Read the model definition and answer for the solid it produces. Units are mm, in the model's axes. Face numbers are marked on the shaded views. Coordinates: 2 decimals unless noted, no trailing zeros. Loops run counter-clockwise (first coordinate to the right, second up) from the corner with the lowest first, then second, coordinate; pieces in that order, holes last. Notation, with made-up numbers: (49, -10) -> (56, -10) arc R19 cw to (56, -5) -> close; hole circle Ø10 at (61, -32). An arc over 180 degrees is marked (long way). Answer as a JSON object with one key per item and string values. Group by question number.
1) Section B-B, the plane z = 32 is taken. Give the vertices of the cut face in (x, y).
2) Section A-A, the plane x = 20 is taken. Give the vertices of the cut face in (y, z).
3) Consider probe 1 along X at (y, z) = (0.5, 147.5); probe 2 along Z at (x, y) = (34.5, -8.5); probe 3 along Z at (x, y) = (16.5, -7). Determine where each line is inside the solid, lowest interval first. Write a range as [from, to].
4) Section C-C, the plane y = 5 is taken. Give the vertices of the cut face in (x, z), plus the area to 3 significant figures.
5) Flat-ended cylindrical pins translate along their axes: P1, Ø24, axis at x = 28, y = 7, coming from the +Z side; P2, Ø18, axis at y = 0, z = 0, coming from the -X side; P3, Ø3, axis at x = 15.5, y = 9.5, coming from the +Z side; P4, Ø24, axis at x = 28.5, y = -7, coming from the -Z side. Find the tip coordinate at first contact, or state that the pin passes through.
6) Determine the mould class of the marked faces 1, 2, 3 and 4 for opening direction Z: released by +Z, released by -Z, zero draft, split by the parting line, or undercut.
7) Section D-D, the plane y = -14.5 is taken. Give the vertices of the cut face in (x, z).
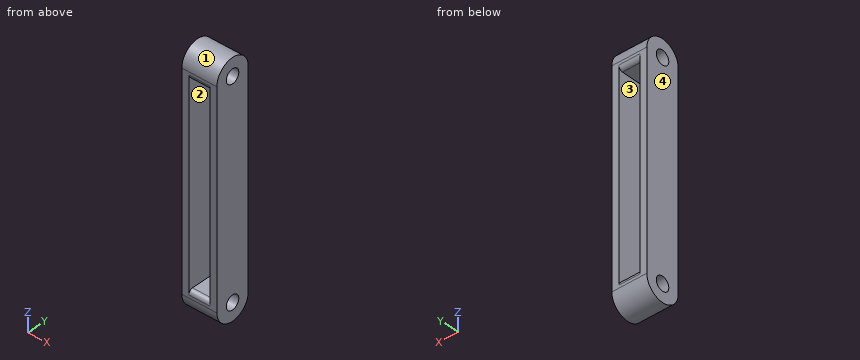
Autodesk Inventor part; units mm, degrees
ref_plane "YZ Plane" through (0, 0, 0) normal (1, 0, 0) x (0, 1, 0)
ref_plane "XZ Plane" through (0, 0, 0) normal (0, 1, 0) x (-1, 0, 0)
ref_plane "XY Plane" through (0, 0, 0) normal (0, 0, 1) x (1, 0, 0)
sketch "Sketch1" plane through (0, 0, 0) normal (1, 0, 0) x (0, 1, 0)
  circle A0 centre (0, 0) radius 25
  line L0 (0, 0) -> (0, 300)
  circle A1 centre (0, 300) radius 25
  circle A2 centre (0, 300) radius 10
  circle A3 centre (0, 0) radius 10
  line L1 (25, 300) -> (25, 0)
  line L2 (-25, 300) -> (-25, 0)
  dimension "d0" = 300
  dimension "d1" = 50
  dimension "d2" = 20
extrude "Extrusion1" add sketch "Sketch1" along normal blind 50
sketch "Sketch2" plane through (0, -25, 0) normal (0, -1, 0) x (1, 0, 0)
  line L0 (0, 0) -> (50, 0)
  line L1 (50, 300) -> (50, 0)
  line L2 (0, 0) -> (50, 0)
  line L3 (50, 0) -> (50, 300)
  line L4 (50, 300) -> (0, 300)
  line L5 (0, 300) -> (0, 0)
  line L6 (10, 10) -> (40, 10)
  line L7 (40, 10) -> (40, 290)
  line L8 (40, 290) -> (10, 290)
  line L9 (10, 290) -> (10, 10)
  dimension "d6" = 10
extrude "Extrusion2" cut sketch "Sketch2" against normal through all contours L9 L8 L7 L6
fillet "Fillet1" radius 6 4 edges at (25, 25, 290) (25, 25, 10) (25, -25, 10) (25, -25, 290)
properties part number "arm1"
Determined:
{
 "1": {"outline": "(0, -25) -> (10, -25) -> (10, 25) -> (0, 25) -> close; (40, -25) -> (50, -25) -> (50, 25) -> (40, 25) -> close"},
 "2": {"outline": "(-25, 0) arc R25 ccw to (25, 0) -> (25, 4) arc R6 ccw to (19, 10) -> (-19, 10) arc R6 ccw to (-25, 4) -> close; (-25, 296) arc R6 ccw to (-19, 290) -> (19, 290) arc R6 ccw to (25, 296) -> (25, 300) arc R25 ccw to (-25, 300) -> close; hole circle Ø20 at (0, 0); hole circle Ø20 at (0, 300)"},
 "3": {"probe 1": "[0, 10], [40, 50]", "probe 2": "[-23.51, -5.27], [5.27, 10], [290, 294.73], [305.27, 323.51]", "probe 3": "[-24, -7.14], [7.14, 10], [290, 292.86], [307.14, 324]"},
 "4": {"outline": "(0, -24.49) -> (50, -24.49) -> (50, -8.66) -> (0, -8.66) -> close; (0, 8.66) -> (50, 8.66) -> (50, 291.34) -> (0, 291.34) -> close; (0, 308.66) -> (50, 308.66) -> (50, 324.49) -> (0, 324.49) -> close; hole (10, 10) -> (40, 10) -> (40, 290) -> (10, 290) -> close", "area": "7,320 mm²"},
 "5": {"P1": "z = 325", "P2": "through", "P3": "z = 323.69", "P4": "z = -25"},
 "6": {"face 1": "released by +Z", "face 2": "undercut", "face 3": "undercut", "face 4": "zero draft"},
 "7": {"outline": "(0, -20.37) -> (50, -20.37) -> (50, 320.37) -> (0, 320.37) -> close; hole (10, 10) -> (40, 10) -> (40, 290) -> (10, 290) -> close"}
}
